```python
from build123d import *

# Parameters (mm, degrees)
RESSALTO_EXTRUS_O1_DEPTH             = 23
ESCAREADO_PARA_SFHCS_M31_D           = 3.4
ESCAREADO_PARA_SFHCS_M31_CSINK_D     = 6.72
ESCAREADO_PARA_SFHCS_M31_CSINK_ANGLE = 90
CORTE_EXTRUS_O1_DEPTH                = 124.778027129


with BuildPart() as part:
    # Esboço1 → Ressalto-extrusão1 (new body)
    with BuildSketch(Plane(origin=(0, 0, 0), x_dir=(1, 0, 0), z_dir=(0, 1, 0))):
        with BuildLine():
            Line((36.1, -78.056325817), (-36.1, -78.056325817))
            ThreePointArc((-36.1, -78.056325817), (-45.453875584, -73.006473647), (-54.113307426, -66.841229488))
            Line((-54.113307426, -66.841229488), (-66.841229488, -54.113307426))
            ThreePointArc((-66.841229488, -54.113307426), (-86, 0), (-66.841229488, 54.113307426))
            Line((-66.841229488, 54.113307426), (-54.113307426, 66.841229488))
            ThreePointArc((-54.113307426, 66.841229488), (0, 86), (54.113307426, 66.841229488))
            Line((54.113307426, 66.841229488), (66.841229488, 54.113307426))
            ThreePointArc((66.841229488, 54.113307426), (86, 0), (66.841229488, -54.113307426))
            Line((66.841229488, -54.113307426), (54.113307426, -66.841229488))
            ThreePointArc((54.113307426, -66.841229488), (45.453875584, -73.006473647), (36.1, -78.056325817))
        make_face()
    extrude(amount=RESSALTO_EXTRUS_O1_DEPTH)

    # Escareado para SFHCS M31 (through all)
    with Locations(Plane(origin=(0, 23, 0), x_dir=(1, 0, 0), z_dir=(0, 1, 0))):
        with Locations((47.022820183, -64.72135955), (27.361611466, 75.175409663), (-47.022820183, -64.72135955), (-27.361611466, 75.175409663)):
            CounterSinkHole(ESCAREADO_PARA_SFHCS_M31_D / 2, ESCAREADO_PARA_SFHCS_M31_CSINK_D / 2, counter_sink_angle=ESCAREADO_PARA_SFHCS_M31_CSINK_ANGLE)

    # Esboço6 → Corte-extrusão1 (cut, through all)
    with BuildSketch(Plane(origin=(0, 23, 0), x_dir=(1, 0, 0), z_dir=(0, 1, 0))):
        Polygon((-66.841229488, -54.113307426), (-64.012802363, -51.284880301), (-51.284880301, -64.012802363), (-54.113307426, -66.841229488), align=None)
        Polygon((-66.841229488, 54.113307426), (-64.012802363, 51.284880301), (-51.284880301, 64.012802363), (-54.113307426, 66.841229488), align=None)
        Polygon((66.841229488, -54.113307426), (64.012802363, -51.284880301), (51.284880301, -64.012802363), (54.113307426, -66.841229488), align=None)
        Polygon((66.841229488, 54.113307426), (54.113307426, 66.841229488), (51.284880301, 64.012802363), (64.012802363, 51.284880301), align=None)
    extrude(amount=-CORTE_EXTRUS_O1_DEPTH, mode=Mode.SUBTRACT)


solid = part.part
```
Verification items for the finished model (mm, model axes). A direction names the side the tool comes from. Give positions to 0.01 mm unless a question says otherwise; leave off trailing zeros. Write each loop counter-clockwise with the first axis right and the second up, starting at its lowest first coordinate (ties: lowest second). Pieces come first, ordered by that corner, then holes. Notation, with made-up numbers: (57, 52.5) - (114, 52.5) arc R21 cw to (114, 80.5) - close; hole circle Ø1 at (29.25, 86.25). An arc over 180 degrees is marked (long way). Put each result on its own line as item: value.
Q1. Section check B-B on z = 34.5. Record the cut outline in (x, y), and give its area (3 significant figures).
Result:
outline: (-78.78, 0) - (78.78, 0) - (78.78, 23) - (-78.78, 23) - close
area: 3,620 mm2
Q2. Section check C-C on x = -71. Record the cut outline in (y, z), and give its area (3 significant figures).
Result:
outline: (0, -48.53) - (23, -48.53) - (23, 48.53) - (0, 48.53) - close
area: 2,230 mm2
Q3. Section check A-A on y = 19. Record the cut outline in (x, z), and give its area (3 significant figures).
Result:
outline: (-66.84, -54.11) - (-64.01, -51.28) - (-51.28, -64.01) - (-54.11, -66.84) arc R86 ccw to (54.11, -66.84) - (51.28, -64.01) - (64.01, -51.28) - (66.84, -54.11) arc R86 ccw to (66.84, 54.11) - (64.01, 51.28) - (51.28, 64.01) - (54.11, 66.84) arc R86 ccw to (36.1, 78.06) - (-36.1, 78.06) arc R86 ccw to (-54.11, 66.84) - (-51.28, 64.01) - (-64.01, 51.28) - (-66.84, 54.11) arc R86 ccw to start; hole circle Ø3.4 at (-47.02, 64.72); hole circle Ø3.4 at (-27.36, -75.18); hole circle Ø3.4 at (27.36, -75.18); hole circle Ø3.4 at (47.02, 64.72)
area: 22,500 mm2
Q4. Mould release check, pull along X, two halves, no side actions. Record for faces 1 (the face through (45.58, 11.34, 72.93)), 2 (the face through (-85.996, 11.339, 0.819)), 3 (the face through (-57.7, 11.7, 57.6)): released by +X, released by -X, zero draft, split by the parting line, or undercut.
Result:
face 1: released by +X
face 2: released by -X
face 3: undercut
Q5. Set-up check for faces 4 (the face through (57.7, 11.7, 57.6)), 5 (the face through (1, 11, 78.056)): record each of +Z, -Z, +X, -X, +Y, -Y from which the full face is reachable in a straight line by a thin tool's end or side.
Result:
face 4: +Y, -Y
face 5: +Z, +X, -X, +Y, -Y
Q6. Depth check by flat-ended pin: P1, Ø1, axis at y = 14, z = 12, coming from the +X side; P2, Ø8, axis at x = 7, y = 14.5, coming from the -Z side; P3, Ø2, axis at x = 27.36, z = -75.18, coming from the +Y side; P4, Ø1.5, axis at y = 9.5, z = 1, coming from the -X side. Enter the tip coordinate at first touch or a pass-through.
Result:
P1: x = 85.23
P2: z = -85.95
P3: through
P4: x = -86
Q7. Scan lines: probe 1 along X at (y, z) = (16, -75.5); probe 2 along X at (y, z) = (8.5, 65); probe 3 along Z at (x, y) = (1, 16). Record each from-to range of solid material in increasing order. Write a range as from..to.
Result:
probe 1: -41.18..-29.03, -25.69..25.69, 29.03..41.18
probe 2: -52.27..-48.7, -45.35..45.35, 48.7..52.27
probe 3: -85.99..78.06
